```python
from build123d import *

# Parameters (mm, degrees)
BOSS_EXTRUDE1_DEPTH = 25.4
SKETCH2_R           = 5.08
CUT_EXTRUDE1_DEPTH  = 3.175
SKETCH3_R           = 2.54
CUT_EXTRUDE2_DEPTH  = 3.175


with BuildPart() as part:
    # Sketch1 → Boss-Extrude1 (new body)
    with BuildSketch(Plane(origin=(0, 0, 0), x_dir=(1, 0, 0), z_dir=(0, 1, 0))):
        Polygon((22.225, 9.525), (22.225, -12.7), (25.4, -12.7), (25.4, 12.7), (-25.4, 12.7), (-25.4, 9.525), align=None)
    extrude(amount=BOSS_EXTRUDE1_DEPTH)

    # Sketch2 → Cut-Extrude1 (cut)
    with BuildSketch(Plane(origin=(25.4, 0, 0), x_dir=(0, 0, -1), z_dir=(1, 0, 0))):
        with Locations((-6.35, 12.7)):
            Circle(SKETCH2_R)
    extrude(amount=-CUT_EXTRUDE1_DEPTH, mode=Mode.SUBTRACT)

    # Sketch3 → Cut-Extrude2 (cut)
    with BuildSketch(Plane.XY.offset(-9.525)):
        with Locations((-12.7, 12.7)):
            Circle(SKETCH3_R)
        with Locations((0, 12.7)):
            Circle(SKETCH3_R)
        with Locations((12.7, 12.7)):
            Circle(SKETCH3_R)
    extrude(amount=-CUT_EXTRUDE2_DEPTH, mode=Mode.SUBTRACT)


solid = part.part
```
Can you work these out from the model? Positions are in its coordinate system, mm. A direction names the side the tool comes from. Coordinates: 2 decimals unless noted, no trailing zeros. Loops run counter-clockwise (first coordinate to the right, second up) from the corner with the lowest first, then second, coordinate; pieces in that order, holes last. Notation, with made-up numbers: (65.25, 1) - (76.25, 1) arc R21 cw to (76.25, 25) - close; hole circle Ø4 at (30, -7). An arc over 180 degrees is marked (long way). Answer as CSV lines item,"result". Start each with the question number.
1) Which directions (+Z, -Z, +X, -X, +Y, -Y) give clear straight access to the entire face, cutting with the end or side of a thin tool? Please do faces 1 (the flat face through (-2, 15, -9.525)), 2 (the cylindrical face through (-14.57, 14.42, -11.09)).
2) Suppose I cut it at A-A (y = 12.7). Please give me the cut outline in (x, z) (3 decimals).
3) Suppose I cut it at C-C (z = 6.35). Please give me the cut outline in (x, y) (3 decimals), plus the area to 3 significant figures.
4) For pin 1 (3 mm diameter, centred on x = 12.7, y = 12.7, fed in from +Z); pin 2 (12 mm diameter, centred on y = 9, z = 10, fed in from -X) (3 decimals), each with a flat end and sliding along its axis, tell me the tip position at first contact or that it passes through.
5) Thinking about a two-plate mould opening in Y: for faces 3 (the flat face through (9, 25.4, -10)), 4 (the flat face through (25.4, 13, 0)), 5 (the cylindrical face through (12.37, 15.22, -11.09)), which applies, pulls with the +Y half, pulls with the -Y half, needs draft (parallel to the pull), parting line crosses it, or undercut?
6) Suppose I cut it at B-B (x = 12.7). Please give me the cut outline in (y, z) (3 decimals).
7) I need wall thicknesses on line 1 (Y direction, x = 0, z = -11.2); line 2 (Z direction, x = -9, y = 24) (3 decimals); line 3 (Y direction, x = 23.1, z = 6.35). Which ranges of each line are inside material? Lowest first, please. Write a range as from..to.
8) Suppose I cut it at D-D (y = 16.75). Please give me the cut outline in (x, z) (3 decimals).
Check result:
1,face 1,"+Z, -X, +Y, -Y"
1,face 2,"+Z, -Z"
2,outline,"(-25.4, -12.7) - (-15.24, -12.7) - (-15.24, -9.525) - (-25.4, -9.525) - close; (-10.16, -12.7) - (-2.54, -12.7) - (-2.54, -9.525) - (-10.16, -9.525) - close; (2.54, -12.7) - (10.16, -12.7) - (10.16, -9.525) - (2.54, -9.525) - close; (15.24, -12.7) - (25.4, -12.7) - (25.4, 1.27) - (22.225, 1.27) - (22.225, -9.525) - (15.24, -9.525) - close; (22.225, 11.43) - (25.4, 11.43) - (25.4, 12.7) - (22.225, 12.7) - close"
3,outline,"(22.225, 0) - (25.4, 0) - (25.4, 7.62) - (22.225, 7.62) - close; (22.225, 17.78) - (25.4, 17.78) - (25.4, 25.4) - (22.225, 25.4) - close"
3,area,"48.4 mm²"
4,pin 1,"passes through"
4,pin 2,"stops at x = 22.225"
5,face 3,"pulls with the +Y half"
5,face 4,"needs draft"
5,face 5,"undercut"
6,outline,"(0, -12.7) - (10.16, -12.7) - (10.16, -9.525) - (0, -9.525) - close; (15.24, -12.7) - (25.4, -12.7) - (25.4, -9.525) - (15.24, -9.525) - close"
7,line 1,"y = 0..10.16, 15.24..25.4"
7,line 2,"z = -12.7..-9.525"
7,line 3,"y = 0..7.62, 17.78..25.4"
8,outline,"(-25.4, -12.7) - (25.4, -12.7) - (25.4, 3.283) - (22.225, 3.283) - (22.225, -9.525) - (-25.4, -9.525) - close; (22.225, 9.417) - (25.4, 9.417) - (25.4, 12.7) - (22.225, 12.7) - close"
